Drawing for the job (mm, zero at the part's lowest x, y, z). A direction names the side the tool comes from. Give positions to 0.01 mm unless a question says otherwise; leave off trailing zeros. Write each loop counter-clockwise with the first axis right and the second up, starting at its lowest first coordinate (ties: lowest second). Pieces come first, ordered by that corner, then holes. Notation, with made-up numbers: (-27.5, -14) - (-13.5, -14) arc R33 cw to (-13.5, 23) - close; hole circle Ø8 at (32.5, 74.25). An arc over 180 degrees is marked (long way). Answer as a JSON object with one key per item and string values. Group by question number.
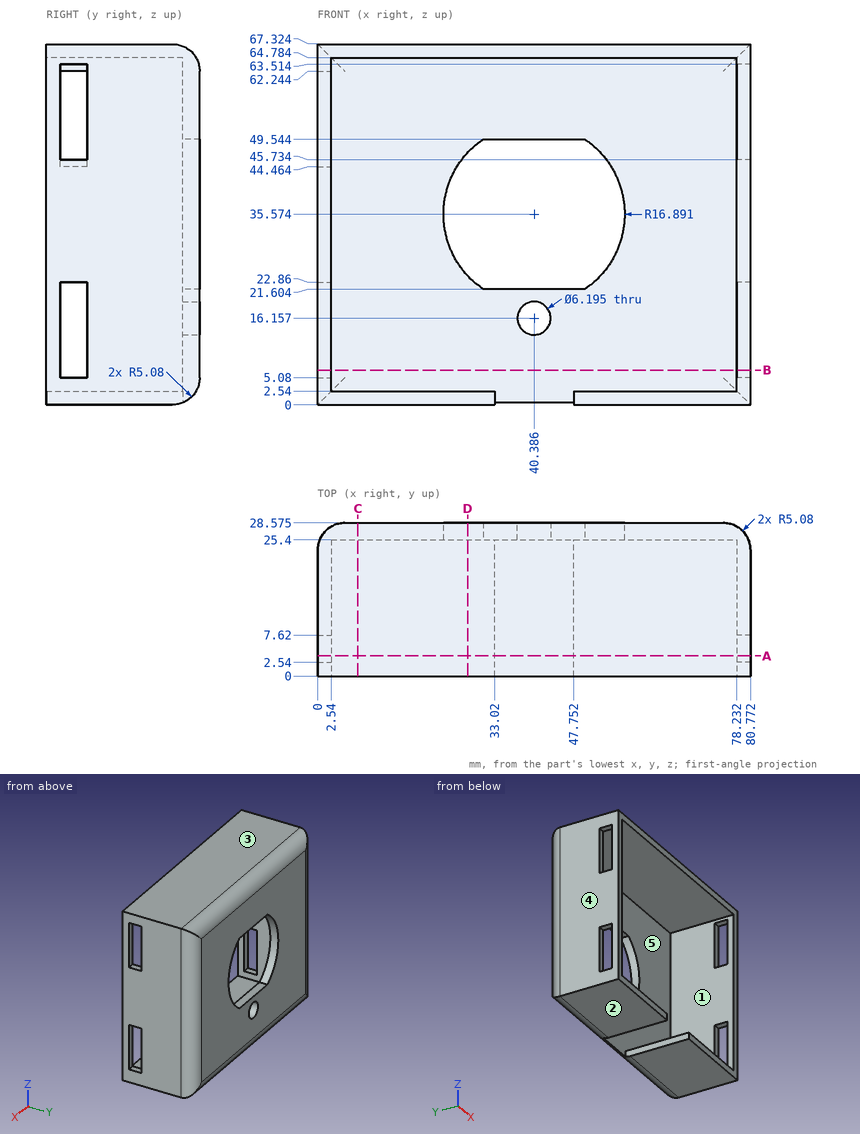
1) Band-saw the part on D-D (x = 28). List the corners of the cut face in (y, z) (1 decimal), plus the area to 3 significant figures.
2) Probe line 1 (Z direction, x = 54, y = 5.5); line 2 (X direction, y = 18.75, z = 42); line 3 (Y direction, x = 68, z = 52) (3 decimals). List the from-to ranges inside material, lowest first.
3) Which spindle directions (+Z, -Z, +X, -X, +Y, -Y) get a long thin tool onto all of the face, cutting with end or side? Do the marked faces 1 and 2. Say none if no direction does.
4) Band-saw the part on B-B (z = 6.5). List the corners of the cut face in (x, y) (3 decimals).
5) Mould opens along Z. For the marked faces 3, 4 and 5 say: pulls with the +Z half, pulls with the -Z half, needs draft (parallel to the pull), parting line crosses it, or undercut.
6) Band-saw the part on C-C (x = 7.5). List the corners of the cut face in (y, z) (3 decimals), plus the area to 3 significant figures.
7) Band-saw the part on A-A (y = 3.75). List the corners of the cut face in (x, z).
8) Drop flat-ended pins along their axis: P1, Ø0.8, axis at x = 0.5, z = 17.5, coming from the +Y side; P2, Ø1.3, axis at x = 79, z = 13.5, coming from the -Y side; P3, Ø2, axis at y = 6, z = 20.5, coming from the -X side; P4, Ø3, axis at x = 80, z = 13, coming from the +Y side. Give the stop position or say it passes through.
Verdict:
{
 "1": {"outline": "(0, 0) - (23.5, 0) arc R5.1 ccw to (28.6, 5.1) - (28.6, 24.1) - (25.4, 24.1) - (25.4, 2.5) - (0, 2.5) - close; (0, 64.8) - (25.4, 64.8) - (25.4, 47.1) - (28.6, 47.1) - (28.6, 62.2) arc R5.1 ccw to (23.5, 67.3) - (0, 67.3) - close", "area": "259 mm2"},
 "2": {"line 1": "0 to 2.54, 64.78 to 67.32", "line 2": "0 to 2.54, 78.23 to 80.77", "line 3": "25.4 to 28.575"},
 "3": {"face 1": "-Y", "face 2": "-Z, +X, -X, +Y, -Y"},
 "4": {"outline": "(0, 0) - (2.54, 0) - (2.54, 2.54) - (0, 2.54) - close; (0, 7.62) - (2.54, 7.62) - (2.54, 25.4) - (78.232, 25.4) - (78.232, 7.62) - (80.772, 7.62) - (80.772, 23.495) arc R5.08 ccw to (75.692, 28.575) - (5.08, 28.575) arc R5.08 ccw to (0, 23.495) - close; (78.232, 0) - (80.772, 0) - (80.772, 2.54) - (78.232, 2.54) - close"},
 "5": {"face 3": "pulls with the +Z half", "face 4": "needs draft", "face 5": "undercut"},
 "6": {"outline": "(0, 0) - (23.495, 0) arc R5.08 ccw to (28.575, 5.08) - (28.575, 62.244) arc R5.08 ccw to (23.495, 67.324) - (0, 67.324) - (0, 64.784) - (25.4, 64.784) - (25.4, 2.54) - (0, 2.54) - close", "area": "332 mm2"},
 "7": {"outline": "(0, 0) - (33.02, 0) - (33.02, 2.54) - (2.54, 2.54) - (2.54, 5.08) - (0, 5.08) - close; (0, 22.86) - (2.54, 22.86) - (2.54, 44.46) - (0, 44.46) - close; (0, 62.24) - (2.54, 62.24) - (2.54, 64.78) - (78.23, 64.78) - (78.23, 63.51) - (80.77, 63.51) - (80.77, 67.32) - (0, 67.32) - close; (47.75, 0) - (80.77, 0) - (80.77, 5.08) - (78.23, 5.08) - (78.23, 2.54) - (47.75, 2.54) - close; (78.23, 22.86) - (80.77, 22.86) - (80.77, 45.73) - (78.23, 45.73) - close"},
 "8": {"P1": "y = 26.38", "P2": "y = 0", "P3": "through", "P4": "y = 27.73"}
}
